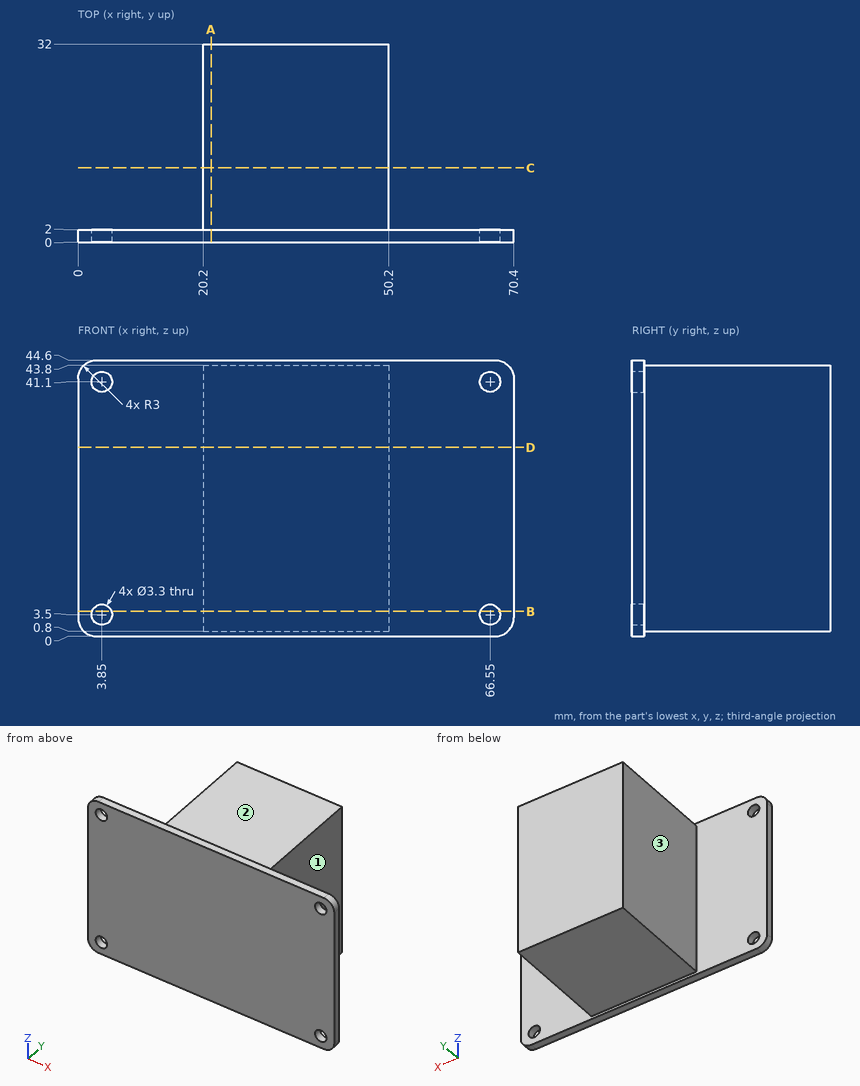
The figure shows three views and two pictorial views of one solid part (mm, origin at its lowest corner). Answer the questions. A direction names the side the tool comes from. Give positions to 0.01 mm unless a question says otherwise; leave off trailing zeros. Write each loop counter-clockwise with the first axis right and the second up, starting at its lowest first coordinate (ties: lowest second). Pieces come first, ordered by that corner, then holes.
Q1. Straight lines are drawn through the part: L1, parallel to X at y = 0.9, z = 41.1; L2, parallel to Z at x = 66, y = 1; L3, parallel to X at y = 24.5, z = 6. For each, find the intervals that lie inside material, in ascending order.
Answer:
L1: x = 0 to 2.2, 5.5 to 64.9, 68.2 to 70.4
L2: z = 0 to 1.94, 5.06 to 39.54, 42.66 to 44.6
L3: x = 20.2 to 50.2
Q2. A tool of negligible diameter and unlimited length cuts with its end or side. For the marked faces 1, 2 and 3, from which of +Z, -Z, +X, -X, +Y, -Y can it reach the whole face along a straight path? Write none if from no direction.
Answer:
face 1: +Z, -Z, +X, +Y
face 2: +Z, +X, -X, +Y
face 3: +Z, -Z, -X, +Y
Q3. The part is cut by section A-A on x = 21.5. Give the vertices of the cut face in (y, z), and give its area (3 significant figures).
Answer:
outline: (0, 0) - (2, 0) - (2, 0.8) - (32, 0.8) - (32, 43.8) - (2, 43.8) - (2, 44.6) - (0, 44.6) - close
area: 1,380 mm2
Q4. The part is cut by section C-C on y = 12. Give the vertices of the cut face in (x, z), and give its area (3 significant figures).
Answer:
outline: (20.2, 0.8) - (50.2, 0.8) - (50.2, 43.8) - (20.2, 43.8) - close
area: 1,290 mm2
Q5. Given pin 1 (10 mm diameter, centred on x = 49, y = 19, fed in from -Z); pin 2 (4 mm diameter, centred on y = 4.5, z = 16.5, fed in from +X); pin 3 (2 mm diameter, centred on y = 16.5, z = 8, fed in from -X); pin 4 (2.5 mm diameter, centred on x = 66.55, z = 3.5, fed in from +Y), each flat-ended and moving along its own axis, determine where each tip first touches the part or whether it passes through.
Answer:
pin 1: stops at z = 0.8
pin 2: stops at x = 50.2
pin 3: stops at x = 20.2
pin 4: passes through
Q6. The part is cut by section B-B on z = 4. Give the vertices of the cut face in (x, y).
Answer:
outline: (0, 0) - (2.28, 0) - (2.28, 2) - (0, 2) - close; (5.42, 0) - (64.98, 0) - (64.98, 2) - (50.2, 2) - (50.2, 32) - (20.2, 32) - (20.2, 2) - (5.42, 2) - close; (68.12, 0) - (70.4, 0) - (70.4, 2) - (68.12, 2) - close
Q7. The part is cut by section D-D on z = 30.5. Give the vertices of the cut face in (x, y).
Answer:
outline: (0, 0) - (70.4, 0) - (70.4, 2) - (50.2, 2) - (50.2, 32) - (20.2, 32) - (20.2, 2) - (0, 2) - close
